```python
from build123d import *

# Parameters (mm, degrees)
F0_W     = 53.4
F0_H     = 55.8
F1_DEPTH = 13.5
F2_R     = 5
F3_R     = 1
F5_D     = 2.4
F5_DEPTH = 4.55
F5_TIP   = 0.7210327428


with BuildPart() as f1:
    # F0 (on Front) → F1 (new body)
    with BuildSketch(Plane.XZ):
        Rectangle(F0_W, F0_H)
    extrude(amount=F1_DEPTH)

    # F2
    f2_edges = [f1.edges().sort_by_distance(p)[0] for p in [
        (-26.7, -6.75, 27.9),
        (26.7, -6.75, 27.9),
        (26.7, -6.75, -27.9),
        (-26.7, -6.75, -27.9),
    ]]
    fillet(f2_edges, radius=F2_R)

    # F3
    f3_edges = [f1.edges().sort_by_distance(p)[0] for p in [
        (0, -13.5, 27.9),
    ]]
    fillet(f3_edges, radius=F3_R)

    # F5
    with Locations(Plane(origin=(0, 0, 0), x_dir=(-1, 0, 0), z_dir=(0, 1, 0))):
        with Locations((-22.5, 22.5), (22.5, 22.5), (22.5, -22.5), (-22.5, -22.5)):
            Hole(F5_D / 2, depth=F5_DEPTH)
            with Locations((0, 0, -(F5_DEPTH + F5_TIP / 2))):  # 118° drill point
                Cone(0, F5_D / 2, F5_TIP, mode=Mode.SUBTRACT)


solid = f1.part
```
Geometry check sheet. Reference: the model listing, model coordinates, mm. A direction names the side the tool comes from. Round coordinates to 2 decimals unless told otherwise and drop trailing zeros. Write each question's results on one line, items separated by ' | '. Start each with the question number.
Q1. Access from +Z, -Z, +X, -X, +Y, -Y to the whole of each face (thin tool, end or side, straight path). Record for faces 1 (the cylindrical face through (-25.27, -6.34, 26.4)), 2 (the cylindrical face through (-23.45, -2.31, 21.77)).
Q2. Release check for a two-part mould opening along X. For faces 3 (the flat face through (0, -13.5, 0)), 4 (the cylindrical face through (25.27, -6.34, 26.4)), 5 (the cylindrical face through (-23.45, -2.31, -23.23)) record: +X half, -X half, draft (parallel to the pull), parting line (faces both ways), or undercut.
Q3. Gauge pin test, flat end, axial feed: P1, Ø1.5, axis at x = -17, z = -6, coming from the +Y side. Record the tip position at first contact, or that the pin passes through.
Q4. Thickness scan on line 1 (X direction, y = -2.9, z = -22.5); line 2 (Z direction, x = 22.5, y = -2.45); line 3 (Z direction, x = -23.5, y = -5.5). Record the ranges inside material, lowest first. Write a range as [from, to].
Answers below:
1) face 1: +Z, -X, +Y, -Y | face 2: +Y
2) face 3: draft | face 4: +X half | face 5: undercut
3) P1: stops at y = 0
4) line 1: x = [-26.7, -23.7], [-21.3, 21.3], [23.7, 26.7] | line 2: z = [-27.84, -23.7], [-21.3, 21.3], [23.7, 27.84] | line 3: z = [-27.56, 27.56]
